Geometry: final body of the model. Coordinates: model frame, mm. A direction names the side the tool comes from. Coordinates: 2 decimals unless noted, no trailing zeros. Write each loop counter-clockwise with the first axis right and the second up, starting at its lowest first coordinate (ties: lowest second). Pieces come first, ordered by that corner, then holes. Notation, with made-up numbers: (-35.5, 52) - (21.5, 52) arc R9 ccw to (21.5, 60) - close; hole circle Ø7 at (49.25, 43.25). An arc over 180 degrees is marked (long way). Put each result on its own line as item: value.
```python
from build123d import *

# Parameters (mm, degrees)
SKETCH1_W            = 79.8
SKETCH1_H            = 32.8
BOSS_EXTRUDE1_DEPTH  = 10
SKETCH3_W            = 79.8
SKETCH3_H            = 19.8
SKETCH3_H_2          = 10.2
SKETCH3_H_3          = 10
BOSS_EXTRUDE3_DEPTH  = 4
BOSS_EXTRUDE4_DEPTH  = 4
SKETCH5_R            = 3.9
BOSS_EXTRUDE5_DEPTH  = 4
FILLET3_R            = 4
FILLET4_R            = 1
BOSS_EXTRUDE9_DEPTH  = 79.8
SKETCH6_R            = 2.25
SKETCH6_R_2          = 2
CUT_EXTRUDE1_DEPTH   = 38.2
BOSS_EXTRUDE10_REACH = 80.553
SKETCH12_R           = 6
SKETCH12_R_2         = 2.25
BOSS_EXTRUDE11_START = 2
SKETCH14_R           = 6
SKETCH14_R_2         = 3.75
BOSS_EXTRUDE11_DEPTH = 2
FILLET5_R            = 0.5


with BuildPart() as part:
    # Sketch1 → Boss-Extrude1 (new body)
    with BuildSketch(Plane.XY):
        Rectangle(SKETCH1_W, SKETCH1_H)
    extrude(amount=BOSS_EXTRUDE1_DEPTH)

    # Sketch3 → Boss-Extrude3 (add)
    with BuildSketch(Plane.XZ.offset(16.4)):
        with Locations((0, -9.9)):
            Rectangle(SKETCH3_W, SKETCH3_H)
        with Locations((0, 15.1)):
            Rectangle(SKETCH3_W, SKETCH3_H_2)
        with Locations((0, 5)):
            Rectangle(SKETCH3_W, SKETCH3_H_3)
    extrude(amount=BOSS_EXTRUDE3_DEPTH)

    # Sketch4 → Boss-Extrude4 (add)
    with BuildSketch(Plane.ZY.offset(39.9)):
        Polygon((10, 16.4), (20.2, -16.4), (20.2, -20.4), (-19.8, -20.4), (-19.8, -16.4), (0, 16.4), align=None)
    boss_extrude4 = extrude(amount=BOSS_EXTRUDE4_DEPTH)

    # Mirror1: Boss-Extrude4 across plane
    add(boss_extrude4.mirror(Plane(origin=(0, 0, 0), x_dir=(0, 0, 1), z_dir=(1, 0, 0))))

    # Sketch5 → Boss-Extrude5 (add)
    with BuildSketch(Plane.XZ.offset(20.4)):
        with BuildLine():
            Line((43.9, 20.2), (43.9, -19.8))
            Line((43.9, -19.8), (55.386672933, -9.72660048))
            Line((55.386672933, -9.72660048), (55.386672933, -9.892664239))
            ThreePointArc((55.386672933, -9.892664239), (65.479337172, 0.2), (55.386672933, 10.292664239))
            Line((55.386672933, 10.292664239), (55.386672933, 10.458727998))
            Line((55.386672933, 10.458727998), (43.9, 20.2))
        make_face()
        with Locations(Location((55.386672933, 0.2, 0), (0, 0, 270))):
            Circle(SKETCH5_R, mode=Mode.SUBTRACT)
    boss_extrude5 = extrude(amount=-BOSS_EXTRUDE5_DEPTH)

    # Mirror2: Boss-Extrude5 across plane
    add(boss_extrude5.mirror(Plane(origin=(0, 0, 0), x_dir=(0, 0, 1), z_dir=(1, 0, 0))))

    # Fillet3
    # the kernel refuses this fillet: 4 mm, written as the material it adds along each edge
    with BuildSketch(Plane(origin=(43.9, -16.4, 30.2), x_dir=(1, 0, 0), z_dir=(0, 0, -1))) as fillet3_piece_1_section:
        with BuildLine():
            CenterArc((FILLET3_R, -FILLET3_R), FILLET3_R, 90, 90)
            Line((0, -FILLET3_R), (0, 0))
            Line((0, 0), (FILLET3_R, 0))
        make_face()
    fillet3_piece_1 = extrude(amount=60, mode=Mode.PRIVATE)
    fillet3_piece_1 = split(fillet3_piece_1, bisect_by=Plane(origin=(54.225128719, -15.491118341, 11.44377547), z_dir=(-0.6467845633993831, 0, -0.7626727532489078)), keep=Keep.TOP, mode=Mode.PRIVATE)
    fillet3_piece_1 = split(fillet3_piece_1, bisect_by=Plane(origin=(54.366477736, -15.491118341, -10.621275019), z_dir=(-0.659340550917199, 0, 0.7518444240108485)), keep=Keep.TOP, mode=Mode.PRIVATE)
    fillet3_piece_1 = split(fillet3_piece_1, bisect_by=Plane(origin=(44.781661859, -6.837280787, -14.027382914), z_dir=(0, -0.5167969163836084, 0.8561080231001189)), keep=Keep.TOP, mode=Mode.PRIVATE)
    fillet3_piece_1 = split(fillet3_piece_1, bisect_by=Plane(origin=(44.781661859, -9.930876549, 18.18826039), z_dir=(0, -0.29694857943139136, -0.9548934711127094)), keep=Keep.TOP, mode=Mode.PRIVATE)
    add(fillet3_piece_1)
    with BuildSketch(Plane(origin=(-43.9, -16.4, 30.2), x_dir=(-1, 0, 0), z_dir=(0, 0, -1))) as fillet3_piece_2_section:
        with BuildLine():
            CenterArc((FILLET3_R, FILLET3_R), FILLET3_R, 180, 90)
            Line((0, FILLET3_R), (0, 0))
            Line((0, 0), (FILLET3_R, 0))
        make_face()
    fillet3_piece_2 = extrude(amount=60, mode=Mode.PRIVATE)
    fillet3_piece_2 = split(fillet3_piece_2, bisect_by=Plane(origin=(-54.366477736, -15.491118341, -10.621275019), z_dir=(0.659340550917199, 0, 0.7518444240108485)), keep=Keep.TOP, mode=Mode.PRIVATE)
    fillet3_piece_2 = split(fillet3_piece_2, bisect_by=Plane(origin=(-44.781661859, -6.837280787, -14.027382914), z_dir=(0, -0.5167969163836084, 0.8561080231001189)), keep=Keep.TOP, mode=Mode.PRIVATE)
    fillet3_piece_2 = split(fillet3_piece_2, bisect_by=Plane(origin=(-54.225128719, -15.491118341, 11.44377547), z_dir=(0.6467845633993831, 0, -0.7626727532489078)), keep=Keep.TOP, mode=Mode.PRIVATE)
    fillet3_piece_2 = split(fillet3_piece_2, bisect_by=Plane(origin=(-44.781661859, -9.930876549, 18.18826039), z_dir=(0, -0.29694857943139136, -0.9548934711127094)), keep=Keep.TOP, mode=Mode.PRIVATE)
    add(fillet3_piece_2)

    # Fillet4
    fillet4_edges = [part.edges().sort_by_distance(p)[0] for p in [
        (0, -16.4, 0),
    ]]
    fillet(fillet4_edges, radius=FILLET4_R)

    # Sketch11 → Boss-Extrude9 (add)
    with BuildSketch(Plane(origin=(-39.9, 0, 0), x_dir=(0, 0, -1), z_dir=(1, 0, 0))):
        Polygon((-20.2, -16.4), (-10, -16.4), (-10, 16.4), align=None)
    extrude(amount=BOSS_EXTRUDE9_DEPTH)

    # Sketch6 → Cut-Extrude1 (cut)
    with BuildSketch(Plane(origin=(0, 0, 0), x_dir=(-1, 0, 0), z_dir=(0, 0, -1))):
        with Locations((-12.45, 0.25)):
            Circle(SKETCH6_R)
        with Locations(Location((12.45, 0.25, 0), (0, 0, 90))):
            Circle(SKETCH6_R)
        with Locations((34.45, 0.2)):
            Circle(SKETCH6_R_2)
        with Locations(Location((-34.45, 0.2, 0), (0, 0, 90))):
            Circle(SKETCH6_R_2)
    extrude(amount=-CUT_EXTRUDE1_DEPTH, mode=Mode.SUBTRACT)

    # Boss-Extrude10: up to this plane
    boss_extrude10_end = Plane(origin=(-43.9, 16.4, 10), z_dir=(0, -0.29694857943139136, -0.9548934711127095))
    # Sketch12 → Boss-Extrude10 (add, up to the surface)
    with BuildSketch(Plane(origin=(0, 0, 18.5), x_dir=(-1, 0, 0), z_dir=(0, 0, -1)), mode=Mode.PRIVATE) as boss_extrude10_sk1:
        with Locations(Location((12.45, 0.25, 0), (0, 0, 270))):
            Circle(SKETCH12_R)
        with Locations((12.45, 0.25)):
            Circle(SKETCH12_R_2, mode=Mode.SUBTRACT)
    boss_extrude10_tool1 = split(extrude(boss_extrude10_sk1.sketch, amount=BOSS_EXTRUDE10_REACH, mode=Mode.PRIVATE), bisect_by=boss_extrude10_end, keep=Keep.BOTH, mode=Mode.PRIVATE)
    add(boss_extrude10_tool1.solids().sort_by_distance((-12.45, 6.080294, 18.5))[0])
    # Sketch12 → Boss-Extrude10 (add, up to the surface)
    with BuildSketch(Plane(origin=(0, 0, 18.5), x_dir=(-1, 0, 0), z_dir=(0, 0, -1)), mode=Mode.PRIVATE) as boss_extrude10_sk2:
        with Locations(Location((-12.45, 0.25, 0), (0, 0, 270))):
            Circle(SKETCH12_R)
        with Locations((-12.45, 0.25)):
            Circle(SKETCH12_R_2, mode=Mode.SUBTRACT)
    boss_extrude10_tool2 = split(extrude(boss_extrude10_sk2.sketch, amount=BOSS_EXTRUDE10_REACH, mode=Mode.PRIVATE), bisect_by=boss_extrude10_end, keep=Keep.BOTH, mode=Mode.PRIVATE)
    add(boss_extrude10_tool2.solids().sort_by_distance((12.45, 6.080294, 18.5))[0])

    # Sketch14 → Boss-Extrude11 (add)
    # profile 1 of 2: a face of its own
    with BuildSketch(Plane.XY.offset(18.5).offset(BOSS_EXTRUDE11_START)):
        with Locations((-12.45, 0.25)):
            Circle(SKETCH14_R)
        with Locations((-12.45, 0.25)):
            Circle(SKETCH14_R_2, mode=Mode.SUBTRACT)
    # profile 2 of 2: a face of its own
    with BuildSketch(Plane.XY.offset(18.5).offset(BOSS_EXTRUDE11_START)):
        with Locations((12.45, 0.25)):
            Circle(SKETCH14_R)
        with Locations((12.45, 0.25)):
            Circle(SKETCH14_R_2, mode=Mode.SUBTRACT)
    extrude(amount=-BOSS_EXTRUDE11_DEPTH)

    # Fillet5
    fillet5_edges = [part.edges().sort_by_distance(p)[0] for p in [
        (-12.449991171, 6.25, 13.156402439),
        (12.450008829, 6.25, 13.156402439),
    ]]
    fillet(fillet5_edges, radius=FILLET5_R)


solid = part.part
```
1. Ray query, probe 1 along X at (y, z) = (-19.55, 0.2); probe 2 along Y at (x, z) = (-43, -11); probe 3 along X at (y, z) = (-9.5, -15). Return the intervals inside material, ascending. Write a range as from..to.
Answer below:
probe 1: x = -65.48..-59.29, -51.49..51.49, 59.29..65.48
probe 2: y = -20.4..-1.82
probe 3: x = -43.9..-39.9, 39.9..43.9
2. Set-up query: faces 1 (the flat face through (12.4, -2.2, 18.5)), 2 (the flat face through (-1, -18, 20.2)), 3 (the flat face through (-39.9, -7, -5)). Return all of +Z, -Z, +X, -X, +Y, -Y with unobstructed straight access to the full face (end or side cutting, diameter ignored); none if empty.
Answer below:
face 1: +Z
face 2: +Z, +X, -X, -Y
face 3: -Z, +Y
3. Pin query (flat end, axial travel): pin 1 Ø2 at (x, z) = (-33.5, -11.5) entering from +Y; pin 2 Ø1.5 at (y, z) = (11, 0) entering from -X; pin 3 Ø5 at (x, y) = (-12.45, 0.25) entering from -Z. Return the tip coordinate at first contact, or that it passes through.
Answer below:
pin 1: stops at y = -16.4
pin 2: stops at x = -43.9
pin 3: stops at z = 0
4. Section query A-A (x = -34.45). Return loops of the section in (y, z).
Answer below:
outline: (-20.4, -19.8) - (-16.4, -19.8) - (-16.4, -1) arc R1 cw to (-15.4, 0) - (-1.8, 0) - (-1.8, 15.66) - (-16.4, 20.2) - (-20.4, 20.2) - close; (2.2, 0) - (16.4, 0) - (16.4, 10) - (2.2, 14.42) - close
5. Mould query, pull axis X, two halves, no side actions, for faces 4 (the cylindrical face through (-14.22, -1.14, 9.38)), 5 (the flat face through (-41.86, -0.23, -10.04)), 6 (the cylindrical face through (15.914, -1.186, 19.514)), 7 (the flat face through (43.9, -1, 1)). Classes: +X half, -X half, draft (parallel to the pull), parting line (faces both ways), or undercut.
Answer below:
face 4: undercut
face 5: draft
face 6: undercut
face 7: +X half
6. Section query B-B (z = -7.5). Return loops of the section in (x, y), then the cut area to 3 significant figures.
Answer below:
outline: (-61.91, -20.4) - (61.91, -20.4) - (61.91, -16.4) - (47.9, -16.4) arc R4 cw to (43.9, -12.4) - (43.9, 3.98) - (39.9, 3.98) - (39.9, -16.4) - (-39.9, -16.4) - (-39.9, 3.98) - (-43.9, 3.98) - (-43.9, -12.4) arc R4 cw to (-47.9, -16.4) - (-61.91, -16.4) - close
area: 665 mm²
7. Section query D-D (y = -8.5). Return loops of the section in (x, z), then the cut area to 3 significant figures.
Answer below:
outline: (-43.9, -15.03) - (-39.9, -15.03) - (-39.9, 0) - (39.9, 0) - (39.9, -15.03) - (43.9, -15.03) - (43.9, 17.74) - (-43.9, 17.74) - close
area: 1,680 mm²
8. Section query C-C (y = 11). Return loops of the section in (x, z), then the cut area to 3 significant figures.
Answer below:
outline: (-43.9, -3.26) - (-39.9, -3.26) - (-39.9, 0) - (39.9, 0) - (39.9, -3.26) - (43.9, -3.26) - (43.9, 11.68) - (-43.9, 11.68) - close
area: 1,050 mm²
